Part model, mm, in its own coordinate system. Face numbers are marked on the shaded views. A direction names the side the tool comes from. Round coordinates to 2 decimals unless told otherwise and drop trailing zeros. Loops run counter-clockwise (first coordinate to the right, second up) from the corner with the lowest first, then second, coordinate; pieces in that order, holes last. Notation, with made-up numbers: (12.25, -2.5) -> (16.25, -2.5) arc R20 cw to (16.25, 21.5) -> close; hole circle Ø5 at (73, 17.5). An arc over 180 degrees is marked (long way). Answer as a JSON object with one key per item and string values. Group by question number.
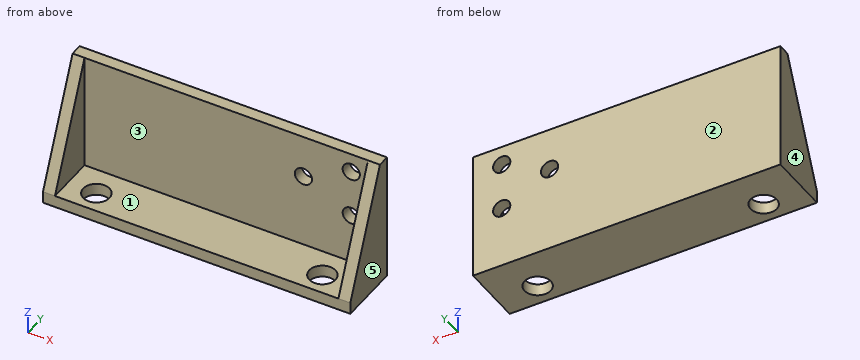
from build123d import *

# Parameters (mm, degrees)
F0_R          = 2.5
F1_DEPTH      = 27
F2_T          = -2.5
F4_DEPTH      = 2.501
F4_DEPTH_BACK = 61.745
F6_D          = 5.5
F7_D          = 3.6


with BuildPart() as f1:
    # F0 (on Top) → F1 (new body)
    with BuildSketch(Plane.XY):
        Polygon((-77.141795, 26.4142), (-45.019795, 26.4142), (-12.897795, 26.4142), (-12.897795, 39.4142), (-77.141795, 39.4142), align=None)
        with Locations((-68.641795, 30.9142)):
            Circle(F0_R, mode=Mode.SUBTRACT)
        with Locations((-21.397795, 30.9142)):
            Circle(F0_R, mode=Mode.SUBTRACT)
        with Locations((-68.641795, 30.9142)):
            Circle(F0_R)
        with Locations((-21.397795, 30.9142)):
            Circle(F0_R)
    extrude(amount=F1_DEPTH)

    # F2
    f2_openings = [f1.faces().sort_by_distance(p)[0] for p in [
        (-45.019795, 32.9142, 27),
        (-45.019795, 26.4142, 13.5),
    ]]
    offset(amount=F2_T, openings=f2_openings)

    # F3 (on face) → F4 (cut, two sides)
    with BuildSketch(Plane.YZ.offset(-74.641795)) as f4_sk:
        Polygon((26.4142, 27), (26.4142, 2.5), (36.9142, 27), align=None)
    extrude(amount=-F4_DEPTH, mode=Mode.SUBTRACT)
    extrude(f4_sk.sketch, amount=F4_DEPTH_BACK, mode=Mode.SUBTRACT)

    # F6 (through all)
    with Locations(Plane(origin=(0, 0, 0), x_dir=(1, 0, 0), z_dir=(0, 0, -1))):
        with Locations((-68.641795, -30.9142), (-21.397795, -30.9142)):
            Hole(F6_D / 2)

    # F7 (through all)
    with Locations(Plane(origin=(0, 39.4142, 0), x_dir=(-1, 0, 0), z_dir=(0, 1, 0))):
        with Locations((18.897795, 13), (18.897795, 23), (28.897795, 18)):
            Hole(F7_D / 2)


solid = f1.part
Item 1: Band-saw the part on A-A, the plane y = 32.75. List the corners of the cut face in (x, z), plus the area to 3 significant figures.
Item 2: Band-saw the part on D-D, the plane y = 36. List the corners of the cut face in (x, z), plus the area to 3 significant figures.
Item 3: Which spindle directions (+Z, -Z, +X, -X, +Y, -Y) get a long thin tool onto all of the face, cutting with end or side? Do the marked faces 1 and 2. Say none if no direction does.
Item 4: Band-saw the part on B-B, the plane z = 18. List the corners of the cut face in (x, y).
Item 5: Drop flat-ended pins along their axis: pin 1 Ø5 at (y, z) = (31.5, 18) entering from -X; pin 2 Ø8 at (x, z) = (-20.5, 15.5) entering from -Y; pin 3 Ø3 at (x, y) = (-59, 30.5) entering from +Z; pin 4 Ø3 at (x, z) = (-18.9, 23) entering from +Y. Give the stop position or say it passes through.
Item 6: Drill centre lines: line 1 (X direction, y = 35.5, z = 9.25); line 2 (Z direction, x = -61, y = 35.75); line 3 (Y direction, x = -69, z = 14.5). Where is each one in solid material? Low to high.
Item 7: Band-saw the part on C-C, the plane x = -59.5. List the corners of the cut face in (y, z).
Item 8: Two-plate mould, pull along X, no slides. Class the marked faces 3, 4 and 5: pulls with the +X half, pulls with the -X half, needs draft (parallel to the pull), parting line crosses it, or undercut.
Entries:
{
 "1": {"outline": "(-77.14, 0) -> (-70.69, 0) -> (-70.69, 2.5) -> (-74.64, 2.5) -> (-74.64, 17.28) -> (-77.14, 17.28) -> close; (-66.59, 0) -> (-23.45, 0) -> (-23.45, 2.5) -> (-66.59, 2.5) -> close; (-19.35, 0) -> (-12.9, 0) -> (-12.9, 17.28) -> (-15.4, 17.28) -> (-15.4, 2.5) -> (-19.35, 2.5) -> close", "area": "214 mm²"},
 "2": {"outline": "(-77.14, 0) -> (-12.9, 0) -> (-12.9, 24.87) -> (-15.4, 24.87) -> (-15.4, 2.5) -> (-74.64, 2.5) -> (-74.64, 24.87) -> (-77.14, 24.87) -> close", "area": "272 mm²"},
 "3": {"face 1": "+Z, -Y", "face 2": "+Z, -Z, +X, -X, +Y"},
 "4": {"outline": "(-77.14, 33.06) -> (-74.64, 33.06) -> (-74.64, 36.91) -> (-30.7, 36.91) -> (-30.7, 39.41) -> (-77.14, 39.41) -> close; (-27.1, 36.91) -> (-15.4, 36.91) -> (-15.4, 33.06) -> (-12.9, 33.06) -> (-12.9, 39.41) -> (-27.1, 39.41) -> close"},
 "5": {"pin 1": "x = -77.14", "pin 2": "y = 36.91", "pin 3": "z = 2.5", "pin 4": "through"},
 "6": {"line 1": "-77.14 to -74.64, -15.4 to -12.9", "line 2": "0 to 2.5", "line 3": "36.91 to 39.41"},
 "7": {"outline": "(26.41, 0) -> (39.41, 0) -> (39.41, 27) -> (36.91, 27) -> (36.91, 2.5) -> (26.41, 2.5) -> close"},
 "8": {"face 3": "undercut", "face 4": "pulls with the -X half", "face 5": "pulls with the +X half"}
}
